The listing builds one solid part. Answer for the finished solid, in the listing's coordinates (mm). Face numbers are marked on the shaded views. A direction names the side the tool comes from. Round coordinates to 2 decimals unless told otherwise and drop trailing zeros. Order: outer loops, then holes, each group sorted by start corner. A loop starts at its lowest first (then second) coordinate and runs counter-clockwise, first axis right, second up. Notation, with made-up numbers: M 20.5,-4 L 67.5,-4 A21 cw 67.5,3 Z; hole C -0.5,49 d3. An arc over 180 degrees is marked long. Put each result on its own line as item: value. Start each with the question number.
1. Which of the six approach directions +Z, -Z, +X, -X, +Y, -Y give full straight-line access (tool end or side, diameter ignored) to the marked faces 4, 5, 6, 7 and 8?
2. The part is cut by section D-D (y = 10.5). Give the vertices of the cut face in (x, z).
3. The part is cut by section B-B (y = 0). Give the vertices of the cut face in (x, z), then the cut area to 3 significant figures.
4. The part is cut by section A-A (z = -1). Give the vertices of the cut face in (x, y).
5. Each of these flat-tipped pins is pushed along its axis until it touches: pin 1 Ø3.5 at (x, y) = (-2, 2) entering from -Z; pin 2 Ø1 at (y, z) = (-3.5, 0.5) entering from -X; pin 3 Ø0.5 at (x, y) = (-6.5, 0.5) entering from -Z. Where does it stop, or does it pass through?
6. The mould has two halves that part along Y. Classify the marked faces 1, 2 and 3: +Y half, -Y half, draft (parallel to the pull), parting line (faces both ways), or undercut.
7. Consider line 1 (X direction, y = -4, z = -2.75); line 2 (Y direction, x = 0.25, z = 1.25). Determine where each line is inside the solid, lowest interval first.
8. The part is cut by section C-C (y = -13). Give the vertices of the cut face in (x, z).
from build123d import *

# Parameters (mm, degrees)
BOSS_EXTRUDE1_DEPTH = 2
BOSS_EXTRUDE2_DEPTH = 0.5
CUT_EXTRUDE1_DEPTH  = 0.1
SKETCH4_W           = 11
SKETCH4_H           = 11
SKETCH4_W_2         = 9
SKETCH4_H_2         = 9
EXTRUDE_THIN1_DEPTH = 6


with BuildPart() as part:
    # Sketch1 → Boss-Extrude1 (new body)
    with BuildSketch(Plane.XY):
        with BuildLine():
            Line((6, 10), (6, -10))
            ThreePointArc((6, -10), (0, -16), (-6, -10))
            Line((-6, -10), (-6, 10))
            ThreePointArc((-6, 10), (0, 16), (6, 10))
        make_face()
    extrude(amount=BOSS_EXTRUDE1_DEPTH)

    # Sketch2 → Boss-Extrude2 (add)
    with BuildSketch(Plane.XY.offset(2)):
        with BuildLine():
            Line((-6, 1), (6, 1))
            ThreePointArc((6, 1), (7, 0), (6, -1))
            Line((6, -1), (-6, -1))
            ThreePointArc((-6, -1), (-7, 0), (-6, 1))
        make_face()
    extrude(amount=BOSS_EXTRUDE2_DEPTH)

    # Sketch3 → Cut-Extrude1 (cut)
    with BuildSketch(Plane.XY.offset(2)):
        Polygon((0, 15), (-2.775609333, 11.00312256), (-1.83190216, 11.00312256), (0, 13.641061671), (1.83190216, 11.00312256), (2.775609333, 11.00312256), align=None)
        Polygon((-2.775609333, -11.00312256), (-1.83190216, -11.00312256), (0, -13.641061671), (1.83190216, -11.00312256), (2.775609333, -11.00312256), (0, -15), align=None)
    extrude(amount=-CUT_EXTRUDE1_DEPTH, mode=Mode.SUBTRACT)

    # Sketch4 → Extrude-Thin1 (add)
    with BuildSketch(Plane(origin=(0, 0, 0), x_dir=(-1, 0, 0), z_dir=(0, 0, -1))):
        Rectangle(SKETCH4_W, SKETCH4_H)
        Rectangle(SKETCH4_W_2, SKETCH4_H_2, mode=Mode.SUBTRACT)
    extrude(amount=EXTRUDE_THIN1_DEPTH)


solid = part.part
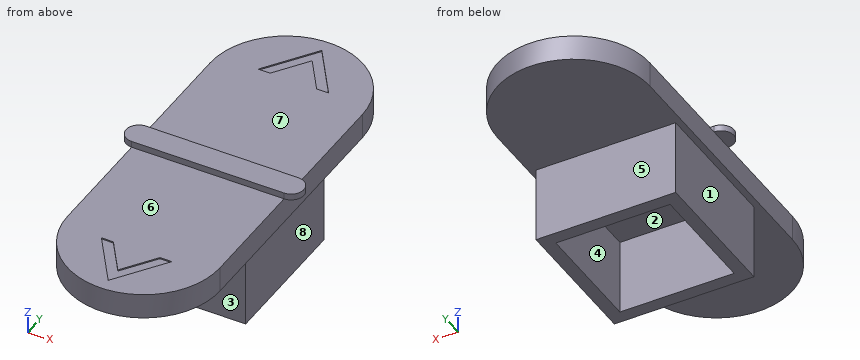
Resolved:
1. face 4: -Z
1. face 5: -Z, +X, -X, +Y
1. face 6: +Z, +X, -X, -Y
1. face 7: +Z, +X, -X, +Y
1. face 8: -Z, +X, +Y, -Y
2. outline: M -5.98,0 L 5.98,0 L 5.98,2 L -5.98,2 Z
3. outline: M -7,2 L -6,2 L -6,0 L -5.5,0 L -5.5,-6 L -4.5,-6 L -4.5,0 L 4.5,0 L 4.5,-6 L 5.5,-6 L 5.5,0 L 6,0 L 6,2 L 7,2 L 7,2.5 L -7,2.5 Z
3. area: 43.0 mm2
4. outline: M -5.5,-5.5 L 5.5,-5.5 L 5.5,5.5 L -5.5,5.5 Z; hole M -4.5,-4.5 L 4.5,-4.5 L 4.5,4.5 L -4.5,4.5 Z
5. pin 1: z = 0
5. pin 2: x = -6
5. pin 3: z = 2
6. face 1: draft
6. face 2: undercut
6. face 3: -Y half
7. line 1: -5.5 to -4.5, 4.5 to 5.5
7. line 2: -15.99 to 15.99
8. outline: M -5.2,0 L 5.2,0 L 5.2,2 L 1.39,2 L 1.39,1.9 L 0.45,1.9 L 0.45,2 L -0.45,2 L -0.45,1.9 L -1.39,1.9 L -1.39,2 L -5.2,2 Z
